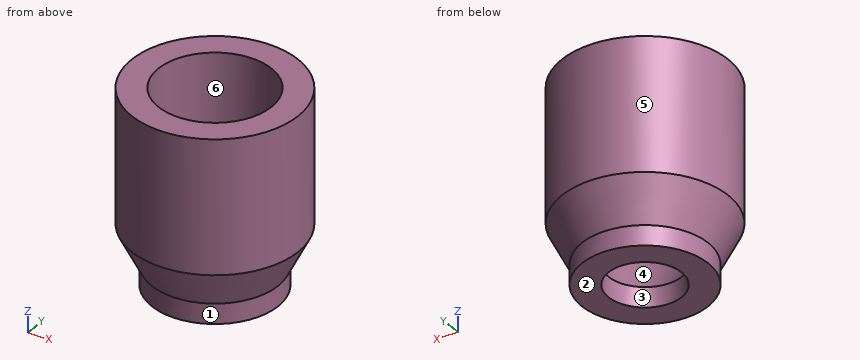
from build123d import *

# Parameters (mm, degrees)
SKETCH1_R           = 4.75
SKETCH2_R           = 6.25
SKETCH1_68_R        = 2.75
SKETCH2_53_R        = 4.25
SKETCH1_69_R        = 4.75
SKETCH1_69_R_2      = 2.75
BOSS_EXTRUDE1_DEPTH = 1.5
SKETCH2_54_R        = 6.25
SKETCH2_54_R_2      = 4.25
BOSS_EXTRUDE2_DEPTH = 10


with BuildPart() as part:
    # Sketch1 → Loft2 section 0
    with BuildSketch(Plane.XY):
        Circle(SKETCH1_R)
    # Sketch2 → Loft2 section 1
    with BuildSketch(Plane.XY.offset(3)):
        Circle(SKETCH2_R)
    loft()

    # Sketch1<68> → Cut-Loft1 section 0
    with BuildSketch(Plane.XY):
        Circle(SKETCH1_68_R)
    # Sketch2<53> → Cut-Loft1 section 1
    with BuildSketch(Plane.XY.offset(3)):
        Circle(SKETCH2_53_R)
    loft(mode=Mode.SUBTRACT)

    # Sketch1<69> → Boss-Extrude1 (add)
    with BuildSketch(Plane.XY):
        Circle(SKETCH1_69_R)
        Circle(SKETCH1_69_R_2, mode=Mode.SUBTRACT)
    extrude(amount=-BOSS_EXTRUDE1_DEPTH)

    # Sketch2<54> → Boss-Extrude2 (add)
    with BuildSketch(Plane.XY.offset(3)):
        Circle(SKETCH2_54_R)
        Circle(SKETCH2_54_R_2, mode=Mode.SUBTRACT)
    extrude(amount=BOSS_EXTRUDE2_DEPTH)


solid = part.part
Model file for the job. Use its own axes, mm. Face numbers are marked on the shaded views. A direction names the side the tool comes from. Round coordinates to 2 decimals unless told otherwise and drop trailing zeros. Loops run counter-clockwise (first coordinate to the right, second up) from the corner with the lowest first, then second, coordinate; pieces in that order, holes last.
1. Drop flat-ended pins along their axis: P1, Ø3.5, axis at x = 0, y = 0, coming from the -Z side; P2, Ø1, axis at x = 3, z = 7.5, coming from the -Y side; P3, Ø4, axis at x = -3.5, z = 2.5, coming from the +Y side; P4, Ø3, axis at x = 2, z = 11, coming from the -Y side. Give the stop position or say it passes through.
Check values:
P1: passes through
P2: stops at y = -5.73
P3: stops at y = 6.05
P4: stops at y = -6.23
2. Band-saw the part on A-A, the plane z = 10.25. List the corners of the cut face in (x, y).
Check values:
outline: circle Ø12.5 at (0, 0); hole circle Ø8.5 at (0, 0)
3. Mould opens along X. For the marked faces 1, 2, 3 and 4 say: +X half, -X half, draft (parallel to the pull), parting line (faces both ways), or undercut.
Check values:
face 1: parting line
face 2: draft
face 3: undercut
face 4: undercut
4. Band-saw the part on B-B, the plane z = -0.5. List the corners of the cut face in (x, y).
Check values:
outline: circle Ø9.5 at (0, 0); hole circle Ø5.5 at (0, 0)
5. Tool access for the marked faces 5 and 6: list every direction of +Z, -Z, +X, -X, +Y, -Y with a clear straight run to the whole face (end or side of a thin tool).
Check values:
face 5: +Z, -Z
face 6: +Z
6. Wall check: probe 1 along Y at (x, z) = (0, 8); probe 2 along Y at (x, z) = (0, -0.8); probe 3 along X at (y, z) = (-3.75, 3.5). Give the ranges that are in metal, low to high.
Check values:
probe 1: y = -6.25 to -4.25, 4.25 to 6.25
probe 2: y = -4.75 to -2.75, 2.75 to 4.75
probe 3: x = -5 to -2, 2 to 5
